```python
from build123d import *

# Parameters (mm, degrees)
BOSS_EXTRUDE1_DEPTH = 3
SKETCH2_W           = 60
SKETCH2_H           = 70
CUT_EXTRUDE1_DEPTH  = 10
SKETCH3_W           = 85
SKETCH3_H           = 50.2
CUT_EXTRUDE2_DEPTH  = 10


with BuildPart() as part:
    # Sketch1 → Boss-Extrude1 (new body)
    with BuildSketch(Plane(origin=(0, 0, 0), x_dir=(0, 0, -1), z_dir=(1, 0, 0))):
        Polygon((-174.354709419, 63.071743487), (125.645290581, 63.071743487), (125.645290581, 35.871743487), (128.645290581, 35.871743487), (128.645290581, -14.128256513), (125.645290581, -14.128256513), (125.645290581, -41.328256513), (-174.354709419, -41.328256513), (-174.354709419, -14.128256513), (-177.354709419, -14.128256513), (-177.354709419, 35.871743487), (-174.354709419, 35.871743487), align=None)
    extrude(amount=BOSS_EXTRUDE1_DEPTH)

    # Sketch2 → Cut-Extrude1 (cut)
    with BuildSketch(Plane(origin=(3, 0, 0), x_dir=(0, 0, -1), z_dir=(1, 0, 0))):
        with Locations((-119.354709419, 10.871743487)):
            Rectangle(SKETCH2_W, SKETCH2_H)
    extrude(amount=-CUT_EXTRUDE1_DEPTH, mode=Mode.SUBTRACT)

    # Sketch3 → Cut-Extrude2 (cut)
    with BuildSketch(Plane(origin=(3, 0, 0), x_dir=(0, 0, -1), z_dir=(1, 0, 0))):
        with Locations((-16.854709419, 10.871743487)):
            Rectangle(SKETCH3_W, SKETCH3_H)
    extrude(amount=-CUT_EXTRUDE2_DEPTH, mode=Mode.SUBTRACT)


solid = part.part
```
Check sheet for the modelled part. Datum: model origin and axes. Units: mm. Give positions to 0.01 mm unless a question says otherwise; leave off trailing zeros. Write each loop counter-clockwise with the first axis right and the second up, starting at its lowest first coordinate (ties: lowest second). Pieces come first, ordered by that corner, then holes. Notation, with made-up numbers: (30, 31.25) -> (51, 31.25) arc R21 ccw to (51, 52.25) -> close; hole circle Ø2 at (82.25, 15.5). An arc over 180 degrees is marked (long way). Use CSV: the item, a comma, the result in double quotes. Start each with the question number.
Q1. Depth check by flat-ended pin: P1, Ø0.9, axis at x = 1, z = -127.5, coming from the +Y side; P2, Ø1.5, axis at x = 2, y = 44, coming from the -Z side; P3, Ø1.5, axis at x = 1, z = -127.5, coming from the -Y side. Enter the tip coordinate at first touch or a pass-through.
Q2. Cross-section at D-D on x = 2.4. Enter the section's corners in (y, z).
Q3. Scan lines: line 1 along Z through (x, y) = (1, 20.5); line 2 along Z through (x, y) = (1.2, -15); line 3 along Z through (x, y) = (0.7, 57). Record each from-to range of solid material in increasing order.
Q4. Cross-section at A-A on y = -4. Enter the section's corners in (x, z).
Q5. Cross-section at C-C on y = -20. Enter the section's corners in (x, z).
Q6. Cross-section at B-B on z = 144. Enter the section's corners in (x, y), and give its area (3 significant figures).
Working result:
1,P1,"stops at y = 35.87"
1,P2,"stops at z = -125.65"
1,P3,"stops at y = -14.13"
2,outline,"(-41.33, -125.65) -> (-14.13, -125.65) -> (-14.13, -128.65) -> (35.87, -128.65) -> (35.87, -125.65) -> (63.07, -125.65) -> (63.07, 174.35) -> (35.87, 174.35) -> (35.87, 177.35) -> (-14.13, 177.35) -> (-14.13, 174.35) -> (-41.33, 174.35) -> close; hole (-24.13, 89.35) -> (45.87, 89.35) -> (45.87, 149.35) -> (-24.13, 149.35) -> close; hole (-14.23, -25.65) -> (35.97, -25.65) -> (35.97, 59.35) -> (-14.23, 59.35) -> close"
3,line 1,"z = -128.65 to -25.65, 59.35 to 89.35, 149.35 to 177.35"
3,line 2,"z = -125.65 to 89.35, 149.35 to 174.35"
3,line 3,"z = -125.65 to 174.35"
4,outline,"(0, -128.65) -> (3, -128.65) -> (3, -25.65) -> (0, -25.65) -> close; (0, 59.35) -> (3, 59.35) -> (3, 89.35) -> (0, 89.35) -> close; (0, 149.35) -> (3, 149.35) -> (3, 177.35) -> (0, 177.35) -> close"
5,outline,"(0, -125.65) -> (3, -125.65) -> (3, 89.35) -> (0, 89.35) -> close; (0, 149.35) -> (3, 149.35) -> (3, 174.35) -> (0, 174.35) -> close"
6,outline,"(0, -41.33) -> (3, -41.33) -> (3, -24.13) -> (0, -24.13) -> close; (0, 45.87) -> (3, 45.87) -> (3, 63.07) -> (0, 63.07) -> close"
6,area,"103 mm^2"
